Geometry: final body of the model. Coordinates: model frame, mm. A direction names the side the tool comes from. Coordinates: 2 decimals unless noted, no trailing zeros. Write each loop counter-clockwise with the first axis right and the second up, starting at its lowest first coordinate (ties: lowest second). Pieces come first, ordered by that corner, then holes. Notation, with made-up numbers: (42.5, 67.25) - (59.5, 67.25) arc R13 ccw to (59.5, 92.25) - close; hole circle Ø1 at (3.5, -20). An arc over 180 degrees is marked (long way). Put each result on its own line as item: value.
```python
from build123d import *

# Parameters (mm, degrees)
F0_W     = 24
F0_H     = 30
F1_DEPTH = 5
F2_W     = 24
F2_H     = 25
F3_DEPTH = 8
F4_R     = 5
F5_W     = 40
F5_H     = 30
F6_DEPTH = 4
F7_W     = 5.5
F7_H     = 11
F8_DEPTH = 2


with BuildPart() as f1:
    # F0 (on Front) → F1 (new body)
    with BuildSketch(Plane.XZ):
        Rectangle(F0_W, F0_H)
    extrude(amount=F1_DEPTH)

    # F2 (on face) → F3 (join)
    with BuildSketch(Plane.XZ.offset(5)):
        with Locations((0, -2.5)):
            Rectangle(F2_W, F2_H)
    extrude(amount=F3_DEPTH)

    # F4
    f4_edges = [f1.edges().sort_by_distance(p)[0] for p in [
        (0, 0, -15),
    ]]
    fillet(f4_edges, radius=F4_R)

    # F5 (on face) → F6 (join)
    with BuildSketch(Plane.XZ.offset(13)):
        Rectangle(F5_W, F5_H)
    extrude(amount=F6_DEPTH)

    # F7 (on face) → F8 (cut)
    with BuildSketch(Plane.XZ.offset(17)):
        with Locations((-12.75, 0)):
            Rectangle(F7_W, F7_H)
        with Locations((12.75, 0)):
            Rectangle(F7_W, F7_H)
    extrude(amount=-F8_DEPTH, mode=Mode.SUBTRACT)


solid = f1.part
```
1. Pin query (flat end, axial travel): pin 1 Ø4 at (y, z) = (-10, -11) entering from -X; pin 2 Ø2.5 at (x, y) = (-3.5, -7.5) entering from +Z; pin 3 Ø4 at (y, z) = (-3.5, 4.5) entering from +X. Return the tip coordinate at first contact, or that it passes through.
Answer below:
pin 1: stops at x = -12
pin 2: stops at z = 10
pin 3: stops at x = 12
2. Section query C-C (y = -15.75). Return loops of the section in (x, z).
Answer below:
outline: (-20, -15) - (20, -15) - (20, 15) - (-20, 15) - close; hole (-15.5, -5.5) - (-10, -5.5) - (-10, 5.5) - (-15.5, 5.5) - close; hole (10, -5.5) - (15.5, -5.5) - (15.5, 5.5) - (10, 5.5) - close
3. Section query D-D (z = -6.75). Return loops of the section in (x, y), then the cut area to 3 significant figures.
Answer below:
outline: (-20, -17) - (20, -17) - (20, -13) - (12, -13) - (12, 0) - (-12, 0) - (-12, -13) - (-20, -13) - close
area: 472 mm²
4. Mould query, pull axis X, two halves, no side actions, for faces 1 (the flat face through (0, 0, 3)), 2 (the flat face through (20, -15, 0)), 3 (the flat face through (10, -16, 0)). Classes: +X half, -X half, draft (parallel to the pull), parting line (faces both ways), or undercut.
Answer below:
face 1: draft
face 2: +X half
face 3: undercut
5. Set-up query: faces 4 (the flat face through (-12, -6, 0)), 5 (the flat face through (0, -17, 0)), 6 (the flat face through (-20, -15, 0)), 7 (the flat face through (0, -9, 10)), 8 (the flat face through (-13, -16, 5.5)). Return all of +Z, -Z, +X, -X, +Y, -Y with unobstructed straight access to the full face (end or side cutting, diameter ignored); none if empty.
Answer below:
face 4: +Z, -Z, -X, +Y
face 5: +Z, -Z, +X, -X, -Y
face 6: +Z, -Z, -X, +Y, -Y
face 7: +Z, +X, -X
face 8: -Y
6. Section query B-B (x = -3). Return loops of the section in (y, z).
Answer below:
outline: (-17, -15) - (-5, -15) arc R5 ccw to (0, -10) - (0, 15) - (-5, 15) - (-5, 10) - (-13, 10) - (-13, 15) - (-17, 15) - close
7. Section query A-A (z = 11.75). Return loops of the section in (x, y), then the cut area to 3 significant figures.
Answer below:
outline: (-20, -17) - (20, -17) - (20, -13) - (-20, -13) - close; (-12, -5) - (12, -5) - (12, 0) - (-12, 0) - close
area: 280 mm²
8. Ray query, probe 1 along Z at (x, y) = (-12, -16); probe 2 along X at (y, z) = (-3.25, 12.5); probe 3 along Y at (x, z) = (17, -2.75). Return the intervals inside material, ascending. Write a range as from..to.
Answer below:
probe 1: z = -15..-5.5, 5.5..15
probe 2: x = -12..12
probe 3: y = -17..-13
